from build123d import *

# Parameters (mm, degrees)
SKETCH_W           = 20
SKETCH_H           = 20
PAD_DEPTH          = 3
POCKET_DEPTH       = 66.886851
POCKET_DEPTH_BACK  = 66.886851
POLARPATTERN_COUNT = 4


with BuildPart() as part:
    # Sketch → Pad (new body)
    with BuildSketch(Plane.XY):
        Rectangle(SKETCH_W, SKETCH_H)
    extrude(amount=PAD_DEPTH)

    # Sketch001 → Pocket (cut, two sides)
    with BuildSketch(Plane.XZ) as pocket_sk:
        with BuildLine():
            Line((10, 0.5), (9.5, 0.552552))
            ThreePointArc((9.5, 0.552552), (7.56125, 2.348555), (5, 3))
            Line((5, 3), (10, 3))
            Line((10, 3), (10, 0.5))
        make_face()
    pocket = extrude(amount=-POCKET_DEPTH, mode=Mode.SUBTRACT) + extrude(pocket_sk.sketch, amount=POCKET_DEPTH_BACK, mode=Mode.SUBTRACT)

    # PolarPattern: Pocket ×4 about axis
    polarpattern_axis = Axis((0, 0, 0), (0, 0, 1))
    for i in range(1, POLARPATTERN_COUNT):
        add(pocket.rotate(polarpattern_axis, i * 360 / POLARPATTERN_COUNT), mode=Mode.SUBTRACT)


solid = part.part
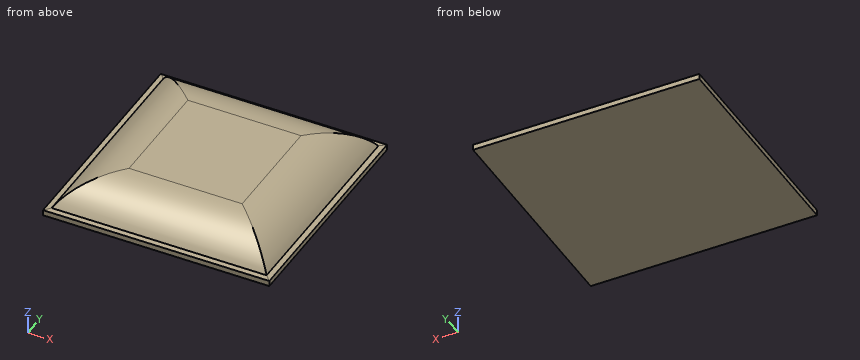
Read the model definition and answer for the solid it produces. Units are mm, in the model's axes. Coordinates: 2 decimals unless noted, no trailing zeros. Loops run counter-clockwise (first coordinate to the right, second up) from the corner with the lowest first, then second, coordinate; pieces in that order, holes last. Notation, with made-up numbers: (40.25, -34.75) -> (92.25, -34.75) arc R25 ccw to (92.25, -13.75) -> close; hole circle Ø6 at (-15.5, 40.25). An arc over 180 degrees is marked (long way). Write item = value, one per line. Start each with the question number.
1) The part is cut by section A-A, the plane x = -3.5. Determine the outline of the cut face in (y, z).
2) The part is cut by section C-C, the plane z = 2.4. Determine the outline of the cut face in (x, y).
3) Find the intervals of material crossed by L1, parallel to Z at x = -5.25, y = -1; L2, parallel to X at y = 0.5, z = 2.55; L3, parallel to Y at x = 7.5, z = 1.65, in increasing order. Write a range as from..to.
4) The part is cut by section D-D, the plane z = 1.1. Determine the outline of the cut face in (x, y), plus the area to 3 significant figures.
Result:
q1.outline = (-10, 0) -> (10, 0) -> (10, 0.5) -> (9.5, 0.55) arc R5.36 ccw to (5, 3) -> (-5, 3) arc R5.36 ccw to (-9.5, 0.55) -> (-10, 0.5) -> close
q2.outline = (-7.46, -7.46) -> (7.46, -7.46) -> (7.46, 7.46) -> (-7.46, 7.46) -> close
q3.L1 = 0..2.99
q3.L2 = -7.15..7.15
q3.L3 = -8.56..8.56
q4.outline = (-9.09, -9.09) -> (9.09, -9.09) -> (9.09, 9.09) -> (-9.09, 9.09) -> close
q4.area = 331 mm²
